```python
from build123d import *

# Parameters (mm, degrees)
EXTRUDE_1_DEPTH = 2


with BuildPart() as part:
    # 草图1 → 凸台-拉伸1 (new body)
    with BuildSketch(Plane.XY):
        Polygon((0, 38.932825237), (4, 38.932825237), (4, 37.482825237), (7.2, 37.482825237), (7.2, 38.932825237), (10.4, 38.932825237), (10.4, 43.032825237), (7.2, 43.032825237), (7.2, 44.482825237), (4, 44.482825237), (4, 43.032825237), (0, 43.032825237), (0, 47.532825237), (20.256410548, 47.532825237), (20.256410548, -21.642820465), (50, -26.602653907), (50, -32.667083917), (46, -32.667083917), (46, -31.217083917), (42.8, -31.217083917), (42.8, -32.667083917), (39.6, -32.667083917), (39.6, -36.767083917), (42.8, -36.767083917), (42.8, -38.217083917), (46, -38.217083917), (46, -36.767083917), (50, -36.767083917), (50, -43.167174763), (20.256410548, -46.217174763), (0, -46.217174763), (0, -41.717174763), (4, -41.717174763), (4, -43.167174763), (7.2, -43.167174763), (7.2, -41.717174763), (10.4, -41.717174763), (10.4, -37.617174763), (7.2, -37.617174763), (7.2, -36.167174763), (4, -36.167174763), (4, -37.617174763), (0, -37.617174763), (0, -28.667174763), (-4, -28.667174763), (-4, -20.667174763), (0, -20.667174763), (0, -11.717174763), (4, -11.717174763), (4, -13.167174763), (7.2, -13.167174763), (7.2, -11.717174763), (10.4, -11.717174763), (10.4, -7.617174763), (7.2, -7.617174763), (7.2, -6.167174763), (4, -6.167174763), (4, -7.617174763), (0, -7.617174763), (0, 21.982825237), (-4, 21.982825237), (-4, 29.982825237), (0, 29.982825237), align=None)
    extrude(amount=EXTRUDE_1_DEPTH)


solid = part.part
```
Geometry check sheet. Reference: the model listing, model coordinates, mm. A direction names the side the tool comes from. Coordinates: 2 decimals unless noted, no trailing zeros. Write each loop counter-clockwise with the first axis right and the second up, starting at its lowest first coordinate (ties: lowest second). Pieces come first, ordered by that corner, then holes. Notation, with made-up numbers: M -3,87.5 L 13,87.5 A7 ccw 13,98.5 Z; hole C 14,-9.75 d6. An arc over 180 degrees is marked long. One line per item, written item: value. Start each with the question number.
(1) Sectioned sample at B-B, the plane x = 34.5. Enter the section's corners in (y, z).
(2) Release check for a two-part mould opening along X. For faces 6 (the face through (2, -41.717, 1)), 7 (the face through (6, -6.167, 1)), 8 (the face through (35.34, -44.67, 0.99)) record: released by +X, released by -X, zero draft, split by the parting line, or undercut.
(3) Sectioned sample at A-A, the plane y = 32.5. Enter the section's corners in (x, z).
(4) Depth check by flat-ended pin: pin 1 (1 mm diameter, centred on y = -35.5, z = 1.5, fed in from +X); pin 2 (1 mm diameter, centred on x = 48, z = 0.5, fed in from +Y); pin 3 (1 mm diameter, centred on y = 3, z = 1, fed in from -X). Enter the tip coordinate at first touch or a pass-through.
(5) Scan lines: line 1 along Y through (x, z) = (9, 0.1); line 2 along Y through (x, z) = (-1.5, 0.3); line 3 along Y through (x, z) = (6, 0.15). Record each from-to range of solid material in increasing order. Write a range as [from, to].
(6) Tool access check on faces 1 (the face through (34.92, -24.09, 0.99)), 2 (the face through (0, 45, 1)), 3 (the face through (10.4, -10, 1)), 4 (the face through (44, -31.217, 1)), 5 (the face through (41, -32.667, 1)). Record the directions out of +Z, -Z, +X, -X, +Y, -Y that give a thin tool (end or side, any length) a straight path to the whole face; none if there is none.
Filled sheet:
1. outline: M -44.76,0 L -24.02,0 L -24.02,2 L -44.76,2 Z
2. face 6: zero draft
2. face 7: undercut
2. face 8: released by +X
3. outline: M 0,0 L 20.26,0 L 20.26,2 L 0,2 Z
4. pin 1: x = 39.6
4. pin 2: y = -26.19
4. pin 3: x = 0
5. line 1: [-46.22, -41.72], [-37.62, -11.72], [-7.62, 38.93], [43.03, 47.53]
5. line 2: [-28.67, -20.67], [21.98, 29.98]
5. line 3: [-46.22, -43.17], [-36.17, -13.17], [-6.17, 37.48], [44.48, 47.53]
6. face 1: +Z, -Z, +X, +Y
6. face 2: +Z, -Z, -X, +Y
6. face 3: +Z, -Z, -X
6. face 4: +Z, -Z
6. face 5: +Z, -Z, +X
